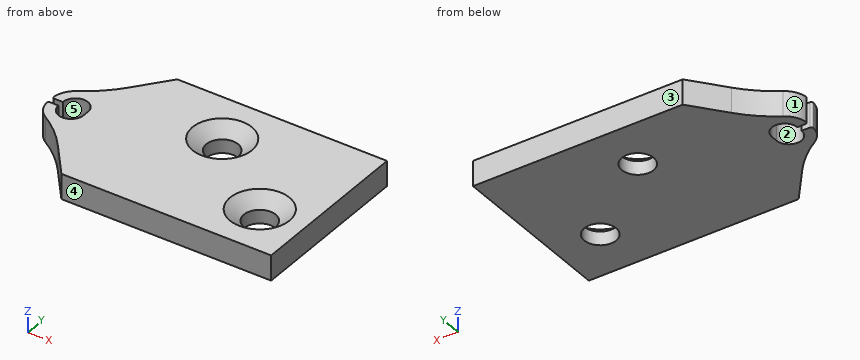
Autodesk Fusion 360 part; units mm, degrees
sketch "Sketch1" plane through (0, 0, 0) normal (0, 0, 1) x (1, 0, 0)
  line L0 (-12.5, 10) -> (12.5, 10)
  line L1 (12.5, 10) -> (12.5, -10)
  line L2 (12.5, -10) -> (-12.5, -10)
  line L3 (-12.5, -10) -> (-12.5, 10)
  dimension "d1" = 20
  dimension "d2" = 25
  dimension "d3" = 12.5
  dimension "d4" = 10
extrude "Extrude1" add sketch "Sketch1" along normal blind 3
sketch "Sketch3" plane through (0, 0, 3) normal (0, 0, 1) x (-1, 0, 0)
  line L0 (12.5, -10) -> (12.5, 10)
  line L1 (12.5, 10) -> (-12.5, 10)
  line L2 (-12.5, 10) -> (-12.5, -10)
  line L3 (-12.5, -10) -> (12.5, -10)
  point P0 (3, -4)
  point P1 (-7, 4)
  dimension "d32" = 5.5
  dimension "d33" = 4
  dimension "d34" = 4
  dimension "d41" = 10
hole "Hole2" at (-3, 4, 3) at (7, -4, 3) direction (0, 0, -1) diameter 3.797 depth 6 tip angle 118 countersink diameter 7.087 countersink angle 100
sketch "Sketch4" plane through (0, 0, 3) normal (0, 0, 1) x (-1, 0, 0)
  circle A0 centre (3, -4) radius 3.5435
  circle A1 centre (-7, 4) radius 3.5435
  line L0 (12.5, 10) -> (-12.5, 10)
  line L1 (-12.5, 10) -> (-12.5, -10)
  line L2 (-12.5, -10) -> (12.5, -10)
  line L3 (12.5, -10) -> (12.5, 10)
  circle A2 centre (18, 0.375) radius 1.5
  circle A3 centre (18, -0.375) radius 1.5
  circle A4 centre (18, 0.375) radius 2.75
  circle A5 centre (18, -0.375) radius 2.75
  line L4 (18, 0.375) -> (17.0157, 0.375)
  line L5 (17.0157, 0.375) -> (17.0157, -0.375)
  line L6 (17.0157, -0.375) -> (18, -0.375)
  line L7 (18, -0.375) -> (18, 0.375)
  line L8 (18, -0.375) -> (24.9519, -0.375)
  line L9 (24.9519, -0.375) -> (24.9519, 0.375)
  line L10 (24.9519, 0.375) -> (18, 0.375)
  line L11 (18, 0.375) -> (18, -0.375)
  line L12 (16.5, 5) -> (16.5, -5)
  line L13 (16.5, 5) -> (12.5, 10)
  line L14 (16.5, -5) -> (12.5, -10)
  dimension "d44" = 3
  dimension "d45" = 3
  dimension "d46" = 5.5
  dimension "d47" = 5.5
  dimension "d48" = 0.75
  dimension "d49" = 0.375
  dimension "d50" = 1.5
  dimension "d51" = 10
  dimension "d52" = 5
  dimension "d55" = 4
extrude "Extrude4" add sketch "Sketch4" against normal blind 3 contours L3 A4 A5 L12 L13 L14 | A4 A5 L12 | A4 A5 L10 L12 | A4 A5 L8 L12 | A4 A5 L12 | A4 A5 L12 | A2 A5 L10 L12 | A3 A4 L8 L12
fillet "Fillet3" radius 15 2 edges at (-16.5, -2.6799, 1.5) (-16.5, 2.6799, 1.5)
fillet "Fillet3" radius 0.25 2 edges at (-20.75, 0.375, 1.5) (-20.75, -0.375, 1.5)
fillet "Fillet3" radius 2 2 edges at (-16.5, 5, 1.5) (-16.5, -5, 1.5)
equation "d49 = ( 0.75 / 2 ) * 1 mm"
Source: CAD feature listing. Evaluate the final solid. Frame: model axes, mm. Face numbers are marked on the shaded views. A direction names the side the tool comes from. Coordinates: 2 decimals unless noted, no trailing zeros. Order: outer loops, then holes, each group sorted by start corner. A loop starts at its lowest first (then second) coordinate and runs counter-clockwise, first axis right, second up. Notation, with made-up numbers: M 35,-34 L 42,-34 A23 ccw 42,-13 Z; hole C -13.5,76.5 d10. An arc over 180 degrees is marked long. Write each question's results on one line, items separated by ' | '. Start each with the question number.
1) Access query for the marked faces 1 and 2. Directions: +Z, -Z, +X, -X, +Y, -Y. A direction counts if a zero-diameter tool reaches every point of the face in a straight line with its end or side. Return the directions, or none.
2) Draft query along Y for the marked faces 3, 4 and 5. Return one class per face: released by +Y, released by -Y, zero draft, split by the parting line, or undercut.
3) Line query: line 1 (Y direction, x = 7, z = 1.25); line 2 (Y direction, x = -3, z = 1.25); line 3 (X direction, y = -4, z = 1.05). Output: solid intervals per line, ascending. Write a range as from..to.
4) Section query B-B (z = 0.65). Give the number of separate pieces and of enclosed holes in the cut face, plus the area to 3 significant figures.
5) Section query A-A (x = 7). Return the cut outline in (y, z), plus the area to 3 significant figures.
6) Contact query for flat-ended pins moving along their axis: pin 1 Ø1 at (x, y) = (-1, -1) entering from -Z; pin 2 Ø1 at (y, z) = (-7.5, 0.5) entering from -X; pin 3 Ø1.1 at (x, z) = (-20, 2) entering from +Y; pin 4 Ø0.6 at (y, z) = (0, 2) entering from -X. Output: stop coordinate, or through.
Answers:
1) face 1: +Z, -Z, -X, +Y | face 2: +Z, -Z
2) face 3: released by +Y | face 4: released by -Y | face 5: undercut
3) line 1: y = -10..-5.9, -2.1..10 | line 2: y = -10..2.1, 5.9..10 | line 3: x = -17.67..5.1, 8.9..12.5
4) separate pieces: 1 | enclosed holes: 2 | area: 555 mm^2
5) outline: M -10,0 L -5.9,0 L -5.9,1.62 L -7.54,3 L -10,3 Z; M -2.1,0 L 10,0 L 10,3 L -0.46,3 L -2.1,1.62 Z | area: 46.3 mm^2
6) pin 1: stops at z = 0 | pin 2: stops at x = -14.9 | pin 3: stops at y = 2.71 | pin 4: stops at x = -16.5
